from build123d import *

# Parameters (mm, degrees)
SKETCH1_R           = 0.4
SKETCH1_W           = 0.52
SKETCH1_H           = 1.1
SKETCH1_H_2         = 1.5
BOSS_EXTRUDE1_DEPTH = 1.5
SKETCH2_W           = 1
SKETCH2_H           = 1.5
BOSS_EXTRUDE2_DEPTH = 1


with BuildPart() as part:
    # Sketch1 → Boss-Extrude1 (new body)
    with BuildSketch(Plane(origin=(0, 0, 0), x_dir=(1, 0, 0), z_dir=(0, 1, 0))):
        Polygon((-9, 33), (9, 33), (9, 0), (4.5, 0), (4.5, 5.5), (-4.5, 5.5), (-4.5, 0), (-9, 0), align=None)
        with Locations(Location((7.62, 1.26, 0), (0, 0, 270))):
            Circle(SKETCH1_R, mode=Mode.SUBTRACT)
        with Locations(Location((7.62, 3.8, 0), (0, 0, 270))):
            Circle(SKETCH1_R, mode=Mode.SUBTRACT)
        with Locations(Location((7.62, 6.34, 0), (0, 0, 270))):
            Circle(SKETCH1_R, mode=Mode.SUBTRACT)
        with Locations(Location((7.62, 8.88, 0), (0, 0, 270))):
            Circle(SKETCH1_R, mode=Mode.SUBTRACT)
        with Locations(Location((7.62, 11.42, 0), (0, 0, 270))):
            Circle(SKETCH1_R, mode=Mode.SUBTRACT)
        with Locations(Location((7.62, 13.96, 0), (0, 0, 270))):
            Circle(SKETCH1_R, mode=Mode.SUBTRACT)
        with Locations(Location((7.62, 16.5, 0), (0, 0, 270))):
            Circle(SKETCH1_R, mode=Mode.SUBTRACT)
        with Locations(Location((7.62, 19.04, 0), (0, 0, 270))):
            Circle(SKETCH1_R, mode=Mode.SUBTRACT)
        with Locations(Location((7.62, 21.58, 0), (0, 0, 270))):
            Circle(SKETCH1_R, mode=Mode.SUBTRACT)
        with Locations(Location((7.62, 24.12, 0), (0, 0, 270))):
            Circle(SKETCH1_R, mode=Mode.SUBTRACT)
        with Locations(Location((7.62, 26.66, 0), (0, 0, 270))):
            Circle(SKETCH1_R, mode=Mode.SUBTRACT)
        with Locations(Location((7.62, 29.2, 0), (0, 0, 270))):
            Circle(SKETCH1_R, mode=Mode.SUBTRACT)
        with Locations(Location((7.62, 31.74, 0), (0, 0, 270))):
            Circle(SKETCH1_R, mode=Mode.SUBTRACT)
        with Locations(Location((-7.62, 31.74, 0), (0, 0, 90))):
            Circle(SKETCH1_R, mode=Mode.SUBTRACT)
        with Locations(Location((-7.62, 29.2, 0), (0, 0, 90))):
            Circle(SKETCH1_R, mode=Mode.SUBTRACT)
        with Locations(Location((-7.62, 26.66, 0), (0, 0, 90))):
            Circle(SKETCH1_R, mode=Mode.SUBTRACT)
        with Locations(Location((-7.62, 24.12, 0), (0, 0, 90))):
            Circle(SKETCH1_R, mode=Mode.SUBTRACT)
        with Locations(Location((-7.62, 21.58, 0), (0, 0, 90))):
            Circle(SKETCH1_R, mode=Mode.SUBTRACT)
        with Locations(Location((-7.62, 19.04, 0), (0, 0, 90))):
            Circle(SKETCH1_R, mode=Mode.SUBTRACT)
        with Locations(Location((-7.62, 16.5, 0), (0, 0, 90))):
            Circle(SKETCH1_R, mode=Mode.SUBTRACT)
        with Locations(Location((-7.62, 13.96, 0), (0, 0, 90))):
            Circle(SKETCH1_R, mode=Mode.SUBTRACT)
        with Locations(Location((-7.62, 11.42, 0), (0, 0, 90))):
            Circle(SKETCH1_R, mode=Mode.SUBTRACT)
        with Locations(Location((-7.62, 8.88, 0), (0, 0, 90))):
            Circle(SKETCH1_R, mode=Mode.SUBTRACT)
        with Locations(Location((-7.62, 6.34, 0), (0, 0, 90))):
            Circle(SKETCH1_R, mode=Mode.SUBTRACT)
        with Locations(Location((-7.62, 3.8, 0), (0, 0, 90))):
            Circle(SKETCH1_R, mode=Mode.SUBTRACT)
        with Locations(Location((-7.62, 1.26, 0), (0, 0, 90))):
            Circle(SKETCH1_R, mode=Mode.SUBTRACT)
        with Locations((5.66, 5.05)):
            Rectangle(SKETCH1_W, SKETCH1_H, mode=Mode.SUBTRACT)
        with Locations((5.66, 1.05)):
            Rectangle(SKETCH1_W, SKETCH1_H_2, mode=Mode.SUBTRACT)
        with Locations((-5.66, 1.05)):
            Rectangle(SKETCH1_W, SKETCH1_H_2, mode=Mode.SUBTRACT)
        with Locations((-5.66, 5.05)):
            Rectangle(SKETCH1_W, SKETCH1_H, mode=Mode.SUBTRACT)
    extrude(amount=-BOSS_EXTRUDE1_DEPTH)

    # Sketch2 → Boss-Extrude2 (add)
    with BuildSketch(Plane(origin=(0, 0, 0), x_dir=(1, 0, 0), z_dir=(0, 1, 0))):
        with Locations((-5.5, 8.53)):
            Rectangle(SKETCH2_W, SKETCH2_H)
        with Locations((5.5, 8.53)):
            Rectangle(SKETCH2_W, SKETCH2_H)
    extrude(amount=BOSS_EXTRUDE2_DEPTH)


solid = part.part
Model file for the job. Use its own axes, mm. A direction names the side the tool comes from. Give positions to 0.01 mm unless a question says otherwise; leave off trailing zeros. Write each loop counter-clockwise with the first axis right and the second up, starting at its lowest first coordinate (ties: lowest second). Pieces come first, ordered by that corner, then holes. Notation, with made-up numbers: M 56,-18.5 L 104,-18.5 A33 cw 104,10.5 Z; hole C 38,-4 d4. An arc over 180 degrees is marked long. One line per item, written item: value. Start each with the question number.
Q1. Probe probe 1 along X at (y, z) = (-0.65, -16.5); probe 2 along X at (y, z) = (-0.7, -2.5); probe 3 along Y at (x, z) = (-0.5, -25). List the from-to ranges inside material, lowest first. Write a range as [from, to].
Q2. Saw through at C-C, the plane z = -11.42. Write the cut outline in (x, y).
Q3. Saw through at D-D, the plane x = -7.62. State how many separate pieces and enclosed holes the cut face has, plus the area to 3 significant figures.
Q4. Drop flat-ended pins along their axis: pin 1 Ø1.5 at (x, y) = (3, 0.5) entering from +Z; pin 2 Ø0.5 at (y, z) = (0.5, -8.5) entering from -X; pin 3 Ø0.8 at (x, y) = (5.5, 0.5) entering from +Z. Give the stop position or say it passes through.
Q5. 3-axis set-ups, long thin cutter, end or side, ignore diameter. For faces 4 (the flat face through (4.5, -1, -3)), 5 (the flat face through (0, -1, -33)), 6 (the flat face through (-5.5, 0.5, -7.78)), 7 (the flat face through (-5.4, -1, -5)): which of +Z, -Z, +X, -X, +Y, -Y reach the whole face in a straight line?
Q6. Saw through at A-A, the plane y = 0.35. Write the cut outline in (x, z).
Q7. Saw through at B-B, the plane z = -2.5. Write the cut outline in (x, y).
Q8. Two-plate mould, pull along Z, no slides. Class faces 1 (the cylindrical face through (7.74, -0.74, -5.96)), 2 (the flat face through (-5.5, 0.5, -9.28)), 3 (the flat face through (-4.5, -1, -3)): +Z half, -Z half, draft (parallel to the pull), parting line (faces both ways), or undercut.
Output values:
1. probe 1: x = [-9, -8.02], [-7.22, 7.22], [8.02, 9]
1. probe 2: x = [-9, -4.5], [4.5, 9]
1. probe 3: y = [-1.5, 0]
2. outline: M -9,-1.5 L -8.02,-1.5 L -8.02,0 L -9,0 Z; M -7.22,-1.5 L 7.22,-1.5 L 7.22,0 L -7.22,0 Z; M 8.02,-1.5 L 9,-1.5 L 9,0 L 8.02,0 Z
3. separate pieces: 14
3. enclosed holes: 0
3. area: 33.9 mm²
4. pin 1: stops at z = -5.5
4. pin 2: stops at x = -6
4. pin 3: stops at z = -7.78
5. face 4: +Z, +Y, -Y
5. face 5: -Z, +X, -X, +Y, -Y
5. face 6: +Z, +X, -X, +Y
5. face 7: +Y, -Y
6. outline: M -6,-9.28 L -5,-9.28 L -5,-7.78 L -6,-7.78 Z; M 5,-9.28 L 6,-9.28 L 6,-7.78 L 5,-7.78 Z
7. outline: M -9,-1.5 L -4.5,-1.5 L -4.5,0 L -9,0 Z; M 4.5,-1.5 L 9,-1.5 L 9,0 L 4.5,0 Z
8. face 1: undercut
8. face 2: -Z half
8. face 3: draft
